from build123d import *

# Parameters (mm, degrees)
SKETCH1_R               = 12.7
SKETCH1_R_2             = 3.175
BOSS_EXTRUDE1_DEPTH     = 2.116666667
SKETCH2_R               = 1.5875
CUT_EXTRUDE1_DEPTH      = 3.116666667
CUT_EXTRUDE1_DEPTH_BACK = 3.116666667


with BuildPart() as part:
    # Sketch1 → Boss-Extrude1 (new body, symmetric)
    with BuildSketch(Plane(origin=(0, 0, 0), x_dir=(1, 0, 0), z_dir=(0, 1, 0))):
        Circle(SKETCH1_R)
        Circle(SKETCH1_R_2, mode=Mode.SUBTRACT)
    extrude(amount=BOSS_EXTRUDE1_DEPTH, both=True)

    # Sketch2 → Cut-Extrude1 (cut, two sides)
    with BuildSketch(Plane(origin=(0, 0, 0), x_dir=(1, 0, 0), z_dir=(0, 1, 0))) as cut_extrude1_sk:
        with Locations((0, 7.9375)):
            Circle(SKETCH2_R)
        with Locations((6.874076643, 3.96875)):
            Circle(SKETCH2_R)
        with Locations((6.874076643, -3.96875)):
            Circle(SKETCH2_R)
        with Locations((0, -7.9375)):
            Circle(SKETCH2_R)
        with Locations((-6.874076643, -3.96875)):
            Circle(SKETCH2_R)
        with Locations((-6.874076643, 3.96875)):
            Circle(SKETCH2_R)
    extrude(amount=CUT_EXTRUDE1_DEPTH, mode=Mode.SUBTRACT)
    extrude(cut_extrude1_sk.sketch, amount=-CUT_EXTRUDE1_DEPTH_BACK, mode=Mode.SUBTRACT)


solid = part.part
The model under review builds one solid part; all positions refer to its coordinate system, in mm. Round coordinates to 2 decimals unless told otherwise and drop trailing zeros. Loops run counter-clockwise (first coordinate to the right, second up) from the corner with the lowest first, then second, coordinate; pieces in that order, holes last. Notation, with made-up numbers: (29.25, 72.5) -> (85.25, 72.5) arc R21 cw to (85.25, 77.5) -> close; hole circle Ø7 at (-10, 68). An arc over 180 degrees is marked (long way). Return JSON: item names as keys, results as strings.
(1) For pin 1 (1.5 mm diameter, centred on y = 1.5, z = -5.5, fed in from +X); pin 2 (1.9 mm diameter, centred on x = 6.87, z = -3.97, fed in from +Y); pin 3 (1 mm diameter, centred on x = -6, y = -0.5, fed in from +Z); pin 4 (1.5 mm diameter, centred on x = -9.5, y = 1, fed in from -Z), all flat-tipped, find the tip position at first contact; note any pin that passes through.
Solved:
{"pin 1": "x = 11.78", "pin 2": "through", "pin 3": "z = 11.45", "pin 4": "z = -9.2"}
(2) Add section D-D on y = 1.75. State how many separate pieces and enclosed holes the cut face has, plus the area to 3 significant figures.
Solved:
{"separate pieces": "1", "enclosed holes": "7", "area": "428 mm2"}
(3) Add section A-A on x = 0. Write out the cut boundary in (y, z) (3 decimals).
Solved:
{"outline": "(-2.117, -12.7) -> (2.117, -12.7) -> (2.117, -9.525) -> (-2.117, -9.525) -> close; (-2.117, -6.35) -> (2.117, -6.35) -> (2.117, -3.175) -> (-2.117, -3.175) -> close; (-2.117, 3.175) -> (2.117, 3.175) -> (2.117, 6.35) -> (-2.117, 6.35) -> close; (-2.117, 9.525) -> (2.117, 9.525) -> (2.117, 12.7) -> (-2.117, 12.7) -> close"}
(4) Add section B-B on z = 0. Write out the cut boundary in (x, y) (3 decimals).
Solved:
{"outline": "(-12.7, -2.117) -> (-3.175, -2.117) -> (-3.175, 2.117) -> (-12.7, 2.117) -> close; (3.175, -2.117) -> (12.7, -2.117) -> (12.7, 2.117) -> (3.175, 2.117) -> close"}
(5) For line 1 (Z direction, x = 0, y = 0.95) (3 decimals); line 2 (X direction, y = 0, z = 4.25); line 3 (Z direction, x = 6.5, y = -1.75), list the stretches that pass through material, from the lowest coordinate up.
Solved:
{"line 1": "-12.7 to -9.525, -6.35 to -3.175, 3.175 to 6.35, 9.525 to 12.7", "line 2": "-11.97 to -8.44, -5.31 to 5.31, 8.44 to 11.97", "line 3": "-10.91 to -5.51, -2.43 to 2.43, 5.51 to 10.91"}
(6) The part is to be moulded in two halves that separate along Z. For faces 1 (the flat face through (3, -2.117, 3)), 2 (the cylindrical face through (5.61, 0.03, 4.93)), 3 (the cylindrical face through (-2.75, 0.03, 12.4)), say which applies: released by +Z, released by -Z, zero draft, split by the parting line, or undercut.
Solved:
{"face 1": "zero draft", "face 2": "undercut", "face 3": "split by the parting line"}
(7) Add section C-C on z = 5. Write out the cut boundary in (x, y), plus the area to 3 significant figures.
Solved:
{"outline": "(-11.67, -2.12) -> (-8.08, -2.12) -> (-8.08, 2.12) -> (-11.67, 2.12) -> close; (-5.67, -2.12) -> (5.67, -2.12) -> (5.67, 2.12) -> (-5.67, 2.12) -> close; (8.08, -2.12) -> (11.67, -2.12) -> (11.67, 2.12) -> (8.08, 2.12) -> close", "area": "78.4 mm2"}
